Autodesk Inventor part; units mm, degrees
ref_plane "YZ Plane" through (0, 0, 0) normal (1, 0, 0) x (0, 1, 0)
ref_plane "XZ Plane" through (0, 0, 0) normal (0, 1, 0) x (-1, 0, 0)
ref_plane "XY Plane" through (0, 0, 0) normal (0, 0, 1) x (1, 0, 0)
sketch "Schizzo1" plane through (0, 0, 0) normal (0, 0, 1) x (1, 0, 0)
  line L0 (-16, 50) -> (16, 50)
  line L1 (-16, 50) -> (-16, 57)
  line L2 (-16, 57) -> (-19, 57)
  line L3 (-19, 57) -> (-19, 0)
  line L4 (16, 50) -> (16, 57)
  line L5 (16, 57) -> (19, 57)
  line L6 (19, 57) -> (19, 0)
  line L7 (-19, 0) -> (19, 0)
  point P0 (0, 0)
  point P1 (0, 0)
  dimension "d2" = 7
  dimension "d3" = 3
  dimension "d4" = 3
  dimension "d5" = 7
  dimension "d6" = 100
  dimension "d7" = 32
  dimension "d8" = 38
revolve "Rivoluzione1" add sketch "Schizzo1" angle 360 about axis through (-19, 0, 0) along (1, 0, 0)
sketch "Schizzo3" plane through (19, 0, 0) normal (1, 0, 0) x (0, 0, -1)
  arc A0 (3, -9.0139) -> (-3, -9.0139) centre (0, 0) ccw
  line L0 (3, -12) -> (-3, -12)
  arc A1 (3, -9.0139) -> (-3, -9.0139) centre (0, 0) ccw
  line L1 (-3, -12) -> (3, -12)
  line L2 (3, -12) -> (3, -9.0139)
  line L3 (-3, -12) -> (-3, -9.0139)
  point P0 (0, 0)
extrude "Estrusione2" cut sketch "Schizzo3" against normal up to next
properties part number "Puleggia minore" material "Alluminio 6061"
Geometry: final body of the model. Coordinates: model frame, mm. A direction names the side the tool comes from. Coordinates: 2 decimals unless noted, no trailing zeros. Order: outer loops, then holes, each group sorted by start corner. A loop starts at its lowest first (then second) coordinate and runs counter-clockwise, first axis right, second up. Notation, with made-up numbers: (68.25, 23) - (120.25, 23) arc R18 cw to (120.25, 47) - close; hole circle Ø8 at (72, 33). An arc over 180 degrees is marked (long way). Return JSON: item names as keys, results as strings. Group by question number.
1. Pin query (flat end, axial travel): pin 1 (2 mm diameter, centred on x = -3, z = -24, fed in from -Y); pin 2 (6 mm diameter, centred on x = -0.5, y = -15, fed in from -Z); pin 3 (1.5 mm diameter, centred on x = -8.5, y = -10, fed in from +Z). Return the tip coordinate at first contact, or that it passes through.
2. Cut plane A-A (x = 10.5). Output: boundary loops of the cut face in (y, z), plus the area to 3 significant figures.
3. Cut plane C-C (y = 37). Output: boundary loops of the cut face in (x, z).
4. Set-up query: faces 4 (the face through (-16, -0.3, -50.4)), 5 (the face through (0, -12, 0)). Return all of +Z, -Z, +X, -X, +Y, -Y with unobstructed straight access to the full face (end or side cutting, diameter ignored); none if empty.
5. Material intervals for line 1 along X through (y, z) = (-51, 23); line 2 along Z through (x, y) = (-8, 0); line 3 along Y through (x, z) = (8, -7), sorted ascending. Write a range as [from, to].
6. Cut plane B-B (z = 0). Output: boundary loops of the cut face in (x, y).
7. Cut plane D-D (z = -20). Output: boundary loops of the cut face in (x, y), plus the area to 3 significant figures.
8. Pull-direction query (X, two-part tool) for faces 1 (the face through (16, -0.3, -50.4)), 2 (the face through (19, -1, -12)), 3 (the face through (-19, -1, -12)); classes: pulls with the +X half, pulls with the -X half, needs draft (parallel to the pull), parting line crosses it, or undercut.
Resolved:
{
 "1": {"pin 1": "stops at y = -44.4", "pin 2": "stops at z = -48.54", "pin 3": "stops at z = 49.14"},
 "2": {"outline": "circle Ø100 at (0, 0); hole (-12, -3) - (-9.01, -3) arc R9.5 ccw (long way) to (-9.01, 3) - (-12, 3) - close", "area": "7,550 mm²"},
 "3": {"outline": "(-19, -43.36) - (-16, -43.36) - (-16, -33.63) - (16, -33.63) - (16, -43.36) - (19, -43.36) - (19, 43.36) - (16, 43.36) - (16, 33.63) - (-16, 33.63) - (-16, 43.36) - (-19, 43.36) - close"},
 "4": {"face 4": "none", "face 5": "+X, -X"},
 "5": {"line 1": "x = [-19, -16], [16, 19]", "line 2": "z = [-50, -9.5], [9.5, 50]", "line 3": "y = [-49.51, -6.42], [6.42, 49.51]"},
 "6": {"outline": "(-19, -57) - (-16, -57) - (-16, -50) - (16, -50) - (16, -57) - (19, -57) - (19, -12) - (-19, -12) - close; (-19, 9.5) - (19, 9.5) - (19, 57) - (16, 57) - (16, 50) - (-16, 50) - (-16, 57) - (-19, 57) - close"},
 "7": {"outline": "(-19, -53.38) - (-16, -53.38) - (-16, -45.83) - (16, -45.83) - (16, -53.38) - (19, -53.38) - (19, 53.38) - (16, 53.38) - (16, 45.83) - (-16, 45.83) - (-16, 53.38) - (-19, 53.38) - close", "area": "3,570 mm²"},
 "8": {"face 1": "undercut", "face 2": "pulls with the +X half", "face 3": "pulls with the -X half"}
}
